Work out the finished part from the listing and answer in its coordinate system (mm). A direction names the side the tool comes from. Round coordinates to 2 decimals unless told otherwise and drop trailing zeros. Write each loop counter-clockwise with the first axis right and the second up, starting at its lowest first coordinate (ties: lowest second). Pieces come first, ordered by that corner, then holes. Notation, with made-up numbers: M 16.5,69 L 75.5,69 A24 cw 75.5,103 Z; hole C -9.75,18.25 d10. An arc over 180 degrees is marked long. One line per item, written item: value. Start each with the question number.
Q1. Find section A-A (z = 0). Write down the section's boundary in (x, y), and give its area (3 significant figures).
Q2. Given pin 1 Ø2 at (y, z) = (-22.5, 23) entering from -X; pin 2 Ø6 at (x, y) = (23.5, -16) entering from +Z; pin 3 Ø8 at (x, y) = (2.5, -8) entering from +Z, each flat-ended and moving along its own axis, determine where each tip first touches the part or whether it passes through.
Q3. Find section B-B (x = 0). Write down the section's boundary in (y, z).
Q4. Consider probe 1 along Z at (x, y) = (0, -15); probe 2 along Z at (x, y) = (0, -5); probe 3 along Y at (x, z) = (-54, -20). Determine where each line is inside the solid, lowest interval first.
Q5. The mould has two halves that part along Z. Classify faces 4 (the cylindrical face through (-62.44, -17.82, 2.75)), 5 (the flat face through (12, -36, -12)), 6 (the cylindrical face through (12.932, -31.81, -5.362)): released by +Z, released by -Z, zero draft, split by the parting line, or undercut.
Q6. Find section D-D (y = -3). Write down the section's boundary in (x, z), and give its area (3 significant figures).
Q7. A tool of negligible diameter and unlimited length cuts with its end or side. For faces 1 (the flat face through (-5.3, -27.5, 11.5)), 2 (the flat face through (12, 0, -12)), 3 (the flat face through (5.3, -10, 11.5)), from which of +Z, -Z, +X, -X, +Y, -Y can it reach the whole face along a straight path? Write none if from no direction.
Q8. Find section C-C (y = -24.5). Write down the section's boundary in (x, z), and give its area (3 significant figures).
from build123d import *

# Parameters (mm, degrees)
F0_R     = 62.5
F1_DEPTH = 36
F2_R     = 5
F3_R     = 12.5
F4_DEPTH = 36.001
F5_R     = 14
F6_DEPTH = 8.5
F7_R     = 14
F8_DEPTH = 10


with BuildPart() as f1:
    # F0 (on Front) → F1 (new body)
    with BuildSketch(Plane.XZ):
        Circle(F0_R)
    extrude(amount=F1_DEPTH)

    # F2
    f2_edges = [f1.edges().sort_by_distance(p)[0] for p in [
        (-62.5, -36, 0),
        (-62.5, 0, 0),
    ]]
    fillet(f2_edges, radius=F2_R)

    # F3 (on face) → F4 (cut, through all)
    with BuildSketch(Plane(origin=(0, 0, 0), x_dir=(-1, 0, 0), z_dir=(0, 1, 0))):
        Circle(F3_R)
    extrude(amount=-F4_DEPTH, mode=Mode.SUBTRACT)

    # F5 (on face) → F6 (cut)
    with BuildSketch(Plane.XZ.offset(36)):
        Circle(F5_R)
    extrude(amount=-F6_DEPTH, mode=Mode.SUBTRACT)

    # F7 (on face) → F8 (cut)
    with BuildSketch(Plane(origin=(0, 0, 0), x_dir=(-1, 0, 0), z_dir=(0, 1, 0))):
        Circle(F7_R)
    extrude(amount=-F8_DEPTH, mode=Mode.SUBTRACT)


solid = f1.part
The answers:
1. outline: M -62.5,-31 A5 ccw -57.5,-36 L -14,-36 L -14,-27.5 L -12.5,-27.5 L -12.5,-10 L -14,-10 L -14,0 L -57.5,0 A5 ccw -62.5,-5 Z; M 12.5,-27.5 L 14,-27.5 L 14,-36 L 57.5,-36 A5 ccw 62.5,-31 L 62.5,-5 A5 ccw 57.5,0 L 14,0 L 14,-10 L 12.5,-10 Z
1. area: 3,520 mm2
2. pin 1: x = -58.5
2. pin 2: z = 59.04
2. pin 3: z = 62.5
3. outline: M -36,-57.5 A5 ccw -31,-62.5 L -5,-62.5 A5 ccw 0,-57.5 L 0,-14 L -10,-14 L -10,-12.5 L -27.5,-12.5 L -27.5,-14 L -36,-14 Z; M -36,14 L -27.5,14 L -27.5,12.5 L -10,12.5 L -10,14 L 0,14 L 0,57.5 A5 ccw -5,62.5 L -31,62.5 A5 ccw -36,57.5 Z
4. probe 1: -62.5 to -12.5, 12.5 to 62.5
4. probe 2: -62.5 to -14, 14 to 62.5
4. probe 3: -36 to 0
5. face 4: split by the parting line
5. face 5: zero draft
5. face 6: undercut
6. outline: C 0,0 d124.17; hole C 0,0 d28
6. area: 11,500 mm2
7. face 1: -Y
7. face 2: +Z, -Z, +X, -X, +Y
7. face 3: +Y
8. outline: C 0,0 d125; hole C 0,0 d25
8. area: 11,800 mm2
